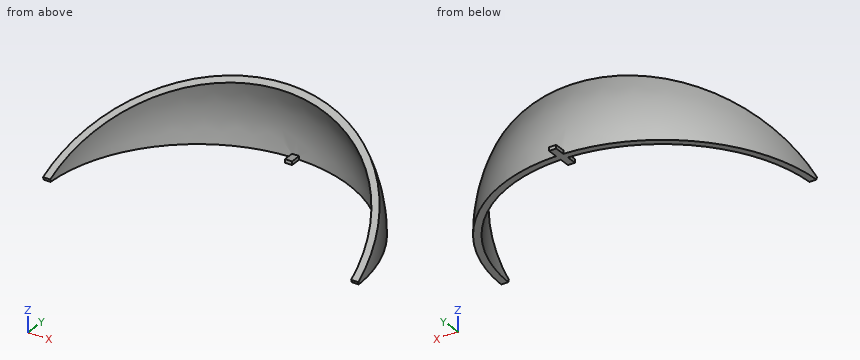
```python
from build123d import *

# Parameters (mm, degrees)
F1_ANGLE      = 30
F2_R          = 3.81
F3_DEPTH      = 113.031
F3_DEPTH_BACK = 113.031
F4_W          = 5.08
F4_H          = 20.3234071666
F5_DEPTH      = 2.54


with BuildPart() as f1:
    # F0 (on Top) → F1 (revolve)
    with BuildSketch(Plane.XY):
        with BuildLine():
            Line((-113.03, 0), (-107.95, 0))
            ThreePointArc((-107.95, 0), (0, 107.95), (107.95, 0))
            Line((107.95, 0), (113.03, 0))
            ThreePointArc((113.03, 0), (0, 113.03), (-113.03, 0))
        make_face()
    revolve(axis=Axis((-53.975, 0, 0), (1, 0, 0)), revolution_arc=F1_ANGLE)

    # F2 (on Right) → F3 (cut, two sides)
    with BuildSketch(Plane.YZ) as f3_sk:
        Circle(F2_R)
    extrude(amount=-F3_DEPTH, mode=Mode.SUBTRACT)
    extrude(f3_sk.sketch, amount=F3_DEPTH_BACK, mode=Mode.SUBTRACT)

    # F4 (on Top) → F5 (join)
    with BuildSketch(Plane.XY):
        with Locations((-1.5036120401, 110.4159437969)):
            Rectangle(F4_W, F4_H)
    extrude(amount=F5_DEPTH)


solid = f1.part
```
Read the model definition and answer for the solid it produces. Units are mm, in the model's axes. Round coordinates to 2 decimals unless told otherwise and drop trailing zeros. Write each loop counter-clockwise with the first axis right and the second up, starting at its lowest first coordinate (ties: lowest second). Pieces come first, ordered by that corner, then holes. Notation, with made-up numbers: (-24, 15) - (3, 15) arc R15 cw to (3, 35) - close; hole circle Ø4 at (84.5, 26.5). An arc over 180 degrees is marked (long way). Use CSV: the item, a comma, the result in double quotes.
Q1. Find section D-D, the plane x = -55. Write down the section's boundary in (y, z).
Values:
outline,"(80.44, 46.44) arc R92.89 cw to (92.89, 0) - (98.75, 0) arc R98.75 ccw to (85.52, 49.37) - close"
Q2. Find section B-B, the plane z = 37. Write down the section's boundary in (x, y), then the cut area to 3 significant figures.
Values:
outline,"(-85.44, 64.09) - (-78.6, 64.09) arc R101.41 cw to (78.6, 64.09) - (85.44, 64.09) arc R106.8 ccw to start"
area,"1,020 mm²"
Q3. Each of these flat-tipped pins is pushed along its axis until it touches: pin 1 Ø1 at (x, z) = (42.5, 29.5) entering from -Y; pin 2 Ø0.8 at (y, z) = (103.5, 1.5) entering from -X; pin 3 Ø1.5 at (x, y) = (-1, 103) entering from +Z; pin 4 Ø12 at (x, y) = (78, 92) entering from +Z. Where does it stop, or does it pass through?
Values:
pin 1,"stops at y = 94.47"
pin 2,"stops at x = -46.3"
pin 3,"stops at z = 48.16"
pin 4,"passes through"
Q4. Find section C-C, the plane y = 56.5. Write down the section's boundary in (x, z).
Values:
outline,"(-97.9, 0) - (-91.98, 0) arc R91.98 cw to (-86.01, 32.62) - (-92.3, 32.62) arc R97.9 ccw to start; (86.01, 32.62) arc R91.98 cw to (91.98, 0) - (97.9, 0) arc R97.9 ccw to (92.3, 32.62) - close"
Q5. Find section A-A, the plane y = 41.5. Write down the section's boundary in (x, z).
Values:
outline,"(-105.14, 0) - (-99.65, 0) arc R99.65 cw to (-96.73, 23.96) - (-102.37, 23.96) arc R105.14 ccw to start; (96.73, 23.96) arc R99.65 cw to (99.65, 0) - (105.14, 0) arc R105.14 ccw to (102.37, 23.96) - close"
Q6. Straight lines are drawn through the part: line 1 along X through (y, z) = (41, 19); line 2 along X through (y, z) = (80, 7.5); line 3 along Y through (x, z) = (70.5, 26). For each, find the intervals that lie inside material, in ascending order.
Values:
line 1,"x = -103.6 to -98.04, 98.04 to 103.6"
line 2,"x = -79.5 to -72.09, 72.09 to 79.5"
line 3,"y = 77.5 to 84.44"
